Here's how the part is built. I have some questions about the finished solid (model axes, mm). Face numbers are marked on the shaded views. A direction names the side the tool comes from. Round coordinates to 2 decimals unless told otherwise and drop trailing zeros. Write each loop counter-clockwise with the first axis right and the second up, starting at its lowest first coordinate (ties: lowest second). Pieces come first, ordered by that corner, then holes. Notation, with made-up numbers: (65, 28) - (124, 28) arc R21 ccw to (124, 58) - close; hole circle Ø7 at (-22, 30.25). An arc over 180 degrees is marked (long way). Write item = value, one per line. Start each with the question number.
Item 1: If I drill on line 1 along X through (y, z) = (2.25, 2.75); line 2 along Y through (x, z) = (0, -4); line 3 along Z through (x, y) = (-4, -2.75), over which ranges is the centre line in solid material (lowest first)? Write a range as [from, to].
Item 2: If we section it at C-C (y = -0.5): Please give me the cut outline in (x, z).
Item 3: For P1, Ø0.6, axis at y = 3, z = 0, coming from the +X side; P2, Ø1.5, axis at y = -1, z = -5.5, coming from the +X side; P3, Ø1, axis at y = 0, z = -3, coming from the +X side, each with a flat end and sliding along its axis, tell me the tip position at first contact or that it passes through.
Item 4: Thinking about a two-plate mould opening in Z: for the marked faces 4, 5 and 6, which applies, pulls with the +Z half, pulls with the -Z half, needs draft (parallel to the pull), parting line crosses it, or undercut?
Item 5: Which directions (+Z, -Z, +X, -X, +Y, -Y) give clear straight access to the entire face, cutting with the end or side of a thin tool? Please do the marked faces 1, 2 and 3.
Item 6: If we section it at B-B (y = 2): Please give me the cut outline in (x, z), and give its area (3 significant figures).
Item 7: If we section it at D-D (y = -2.75): Please give me the cut outline in (x, z), and give its area (3 significant figures).
Item 8: If we section it at A-A (x = 0): Please give me the cut outline in (y, z) (3 decimals).
```python
from build123d import *

# Parameters (mm, degrees)
SKETCH1_R           = 0.75
BOSS_EXTRUDE1_DEPTH = 6.5
SKETCH6_R           = 3.5
BOSS_EXTRUDE4_DEPTH = 2.5
SKETCH7_R           = 5
BOSS_EXTRUDE5_DEPTH = 0.5
SKETCH8_R           = 0.75
CUT_EXTRUDE1_DEPTH  = 3
BOSS_EXTRUDE6_START = 2.5
BOSS_EXTRUDE6_DEPTH = 8.25
CUT_EXTRUDE2_REACH  = 11.5
SKETCH11_R          = 0.375
CUT_EXTRUDE3_START  = 3
SKETCH13_R          = 3
CUT_EXTRUDE3_DEPTH  = 8.5


with BuildPart() as part:
    # Sketch1 → Boss-Extrude1 (new body)
    with BuildSketch(Plane.XY):
        with BuildLine():
            Line((-6, -6.75), (6, -6.75))
            Line((6, -6.75), (3.312648335, 1.129761483))
            ThreePointArc((3.312648335, 1.129761483), (0, 3.5), (-3.312648335, 1.129761483))
            Line((-3.312648335, 1.129761483), (-6, -6.75))
        make_face()
        Circle(SKETCH1_R, mode=Mode.SUBTRACT)
    extrude(amount=-BOSS_EXTRUDE1_DEPTH)

    # Sketch6 → Boss-Extrude4 (add)
    with BuildSketch(Plane.XY):
        Circle(SKETCH6_R)
    extrude(amount=BOSS_EXTRUDE4_DEPTH)

    # Sketch7 → Boss-Extrude5 (add)
    with BuildSketch(Plane.XY.offset(2.5)):
        Circle(SKETCH7_R)
    extrude(amount=BOSS_EXTRUDE5_DEPTH)

    # Sketch8 → Cut-Extrude1 (cut)
    with BuildSketch(Plane.XY.offset(3)):
        Circle(SKETCH8_R)
    extrude(amount=-CUT_EXTRUDE1_DEPTH, mode=Mode.SUBTRACT)

    # Sketch10 → Boss-Extrude6 (add)
    with BuildSketch(Plane.XY.offset(BOSS_EXTRUDE6_START)):
        Polygon((-3, 6), (3, 6), (3, 5.5), (2.5, 5.5), (2.5, 5.05), (3, 5.05), (3, 4.55), (2.5, 4.55), (2.5, 4.1), (3, 4.1), (3, 3.6), (2.5, 3.6), (2.5, 3.15), (3, 3.15), (3, 2.65), (2.5, 2.65), (2.5, 2.2), (3, 2.2), (3, 1.7), (-3, 1.7), (-3, 2.2), (-2.5, 2.2), (-2.5, 2.65), (-3, 2.65), (-3, 3.15), (-2.5, 3.15), (-2.5, 3.6), (-3, 3.6), (-3, 4.1), (-2.5, 4.1), (-2.5, 4.55), (-3, 4.55), (-3, 5.05), (-2.5, 5.05), (-2.5, 5.5), (-3, 5.5), align=None)
    extrude(amount=-BOSS_EXTRUDE6_DEPTH)

    # Sketch11 → Cut-Extrude2 (cut, up to next)
    with BuildSketch(Plane.XY.offset(3), mode=Mode.PRIVATE) as cut_extrude2_sk1:
        with Locations((3.464101615, 2)):
            Circle(SKETCH11_R)
    cut_extrude2_tool1 = extrude(cut_extrude2_sk1.sketch, amount=-CUT_EXTRUDE2_REACH, mode=Mode.PRIVATE) & part.part
    add(cut_extrude2_tool1.solids().sort_by_distance((3.464102, 2, 3))[0], mode=Mode.SUBTRACT)
    # Sketch11 → Cut-Extrude2 (cut, up to next)
    with BuildSketch(Plane.XY.offset(3), mode=Mode.PRIVATE) as cut_extrude2_sk2:
        with Locations((0, -4)):
            Circle(SKETCH11_R)
    cut_extrude2_tool2 = extrude(cut_extrude2_sk2.sketch, amount=-CUT_EXTRUDE2_REACH, mode=Mode.PRIVATE) & part.part
    add(cut_extrude2_tool2.solids().sort_by_distance((0, -4, 3))[0], mode=Mode.SUBTRACT)
    # Sketch11 → Cut-Extrude2 (cut, up to next)
    with BuildSketch(Plane.XY.offset(3), mode=Mode.PRIVATE) as cut_extrude2_sk3:
        with Locations((-3.464101615, 2)):
            Circle(SKETCH11_R)
    cut_extrude2_tool3 = extrude(cut_extrude2_sk3.sketch, amount=-CUT_EXTRUDE2_REACH, mode=Mode.PRIVATE) & part.part
    add(cut_extrude2_tool3.solids().sort_by_distance((-3.464102, 2, 3))[0], mode=Mode.SUBTRACT)

    # Sketch13 → Cut-Extrude3 (cut)
    with BuildSketch(Plane.XY.offset(CUT_EXTRUDE3_START)):
        Circle(SKETCH13_R)
    extrude(amount=-CUT_EXTRUDE3_DEPTH, mode=Mode.SUBTRACT)


solid = part.part
```
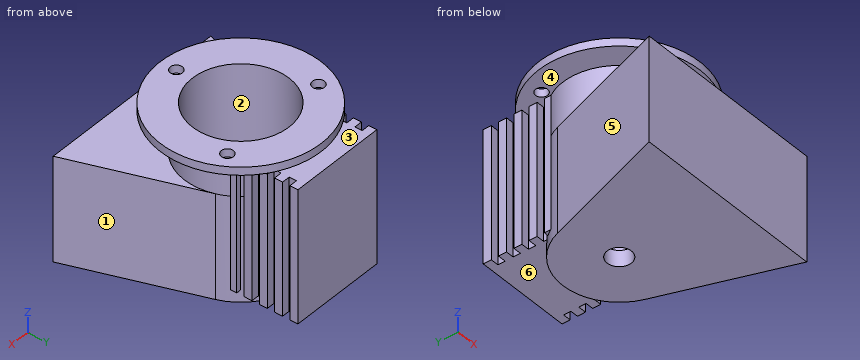
Reply:
q1.line_1 = [-4.47, -3.74], [-3.18, -1.98], [1.98, 3.18], [3.74, 4.47]
q1.line_2 = [-6.75, -3], [3, 6]
q1.line_3 = [-6.5, 0], [2.5, 3]
q2.outline = (-4.97, 2.5) - (-3.46, 2.5) - (-3.46, 0) - (-3.87, 0) - (-3.87, -6.5) - (-0.56, -6.5) - (-0.56, -5.5) - (-2.96, -5.5) - (-2.96, 3) - (-4.97, 3) - close; (0.56, -6.5) - (3.87, -6.5) - (3.87, 0) - (3.46, 0) - (3.46, 2.5) - (4.97, 2.5) - (4.97, 3) - (2.96, 3) - (2.96, -5.5) - (0.56, -5.5) - close
q3.P1 = 3
q3.P2 = 4.29
q3.P3 = 3.87
q4.face_4 = undercut
q4.face_5 = needs draft
q4.face_6 = pulls with the -Z half
q5.face_1 = -Z, +X, +Y
q5.face_2 = +Z
q5.face_3 = +Z, +Y
q6.outline = (-4.58, 2.5) - (-3.84, 2.5) - (-3.84, 3) - (-4.58, 3) - close; (-3.09, 2.5) - (-3, 2.5) - (-3, -5.75) - (-2.87, -5.75) - (-2.87, -6.5) - (2.87, -6.5) - (2.87, -5.75) - (3, -5.75) - (3, 2.5) - (3.09, 2.5) - (3.09, 3) - (2.24, 3) - (2.24, -5.5) - (-2.24, -5.5) - (-2.24, 3) - (-3.09, 3) - close; (3.84, 2.5) - (4.58, 2.5) - (4.58, 3) - (3.84, 3) - close
q6.area = 19.6 mm2
q7.outline = (-4.64, -6.5) - (4.64, -6.5) - (4.64, 0) - (2.17, 0) - (2.17, 2.5) - (4.18, 2.5) - (4.18, 3) - (1.2, 3) - (1.2, -5.5) - (-1.2, -5.5) - (-1.2, 3) - (-4.18, 3) - (-4.18, 2.5) - (-2.17, 2.5) - (-2.17, 0) - (-4.64, 0) - close
q7.area = 54.9 mm2
q8.outline = (-6.75, -6.5) - (-0.75, -6.5) - (-0.75, -5.5) - (-3, -5.5) - (-3, 3) - (-3.625, 3) - (-3.625, 2.5) - (-3.5, 2.5) - (-3.5, 0) - (-6.75, 0) - close; (-5, 2.5) - (-4.375, 2.5) - (-4.375, 3) - (-5, 3) - close; (0.75, -6.5) - (3.5, -6.5) - (3.5, -5.75) - (6, -5.75) - (6, 2.5) - (5, 2.5) - (5, 3) - (3, 3) - (3, -5.5) - (0.75, -5.5) - close
